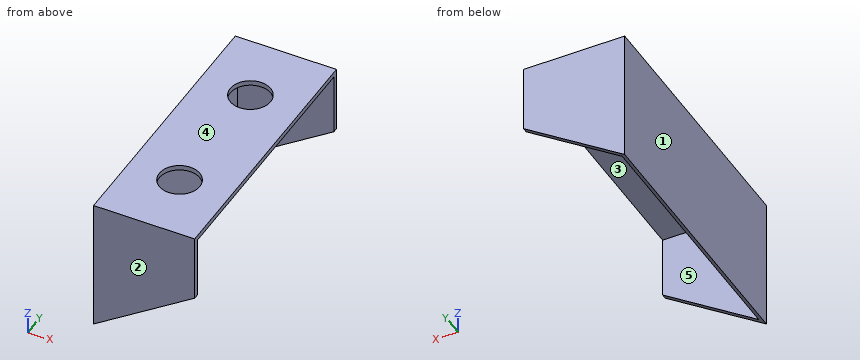
from build123d import *

# Parameters (mm, degrees)
F1_DEPTH = 50.8
F2_R     = 7.62
F3_DEPTH = 50.801
F4_T     = -1.905


with BuildPart() as f1:
    # F0 (on Front) → F1 (new body, symmetric)
    with BuildSketch(Plane.XZ):
        Polygon((0, 50.8), (0, 0), (38.1, 25.4), (38.1, 50.8), align=None)
    extrude(amount=F1_DEPTH, both=True)

    # F2 (on face) → F3 (cut, through all)
    with BuildSketch(Plane.XY.offset(50.8)):
        with Locations((19.05, 25.4)):
            Circle(F2_R)
        with Locations((19.05, -25.4)):
            Circle(F2_R)
    extrude(amount=-F3_DEPTH, mode=Mode.SUBTRACT)

    # F4
    f4_openings = [f1.faces().sort_by_distance(p)[0] for p in [
        (19.05, 0, 12.7),
        (38.1, 0, 38.1),
        (11.43, -25.4, 29.104782),
        (11.43, 25.4, 29.104782),
    ]]
    offset(amount=F4_T, openings=f4_openings)


solid = f1.part
Could you check a few things on this model? Use its own coordinates, in mm. Face numbers are marked on the shaded views. A direction names the side the tool comes from. Give positions to 0.01 mm unless a question says otherwise; leave off trailing zeros. Order: outer loops, then holes, each group sorted by start corner. A loop starts at its lowest first (then second) coordinate and runs counter-clockwise, first axis right, second up. Notation, with made-up numbers: (9.5, 21.5) - (27.5, 21.5) arc R17 ccw to (27.5, 36.5) - close; hole circle Ø3 at (45, 10.25). An arc over 180 degrees is marked (long way). One line per question, with ' | ' between items. Start each with the question number.
Item 1: For the marked faces 4 and 5, which set-ups out of +Z, -Z, +X, -X, +Y, -Y let a thin tool reach every point of the face, with its end or its side?
Item 2: Thinking about a two-plate mould opening in Y: for the marked faces 1, 2 and 3, which applies, pulls with the +Y half, pulls with the -Y half, needs draft (parallel to the pull), parting line crosses it, or undercut?
Item 3: I need wall thicknesses on probe 1 along Y at (x, z) = (19.05, 49.6); probe 2 along Y at (x, z) = (7.5, 46) (3 decimals); probe 3 along X at (y, z) = (25, 49). Which ranges of each line are inside material? Lowest first, please. Write a range as [from, to].
Item 4: I want a section at A-A on x = 19.05. Write out the boundary of the cut face in (y, z) (3 decimals), then the cut area to 3 significant figures.
Item 5: I'm going to push flat-ended pins straight in: pin 1 Ø3 at (x, z) = (34, 20) entering from +Y; pin 2 Ø2 at (y, z) = (15, 44) entering from +X (3 decimals). Where does each tip first touch, or does it pass through?
Item 6: I want a section at D-D on y = -23.5. Write out the boundary of the cut face in (x, z) (3 decimals).
Item 7: I want a section at C-C on x = 31.5. Write out the boundary of the cut face in (y, z) (3 decimals).
Item 8: I want a section at B-B on y = 25.4. Write out the boundary of the cut face in (x, z) (3 decimals).
Verdict:
1) face 4: +Z, +X, -X, +Y, -Y | face 5: -Z, +X
2) face 1: needs draft | face 2: pulls with the -Y half | face 3: undercut
3) probe 1: [-50.8, -33.02], [-17.78, 17.78], [33.02, 50.8] | probe 2: [-50.8, -48.895], [48.895, 50.8] | probe 3: [0, 11.44], [26.66, 38.1]
4) outline: (-50.8, 12.7) - (-48.895, 12.7) - (-48.895, 48.895) - (-33.02, 48.895) - (-33.02, 50.8) - (-50.8, 50.8) - close; (-17.78, 48.895) - (17.78, 48.895) - (17.78, 50.8) - (-17.78, 50.8) - close; (33.02, 48.895) - (48.895, 48.895) - (48.895, 12.7) - (50.8, 12.7) - (50.8, 50.8) - (33.02, 50.8) - close | area: 273 mm^2
5) pin 1: through | pin 2: x = 1.905
6) outline: (0, 0) - (1.905, 1.27) - (1.905, 48.895) - (11.671, 48.895) - (11.671, 50.8) - (0, 50.8) - close; (26.429, 48.895) - (38.1, 48.895) - (38.1, 50.8) - (26.429, 50.8) - close
7) outline: (-50.8, 21) - (-48.895, 21) - (-48.895, 48.895) - (48.895, 48.895) - (48.895, 21) - (50.8, 21) - (50.8, 50.8) - (-50.8, 50.8) - close
8) outline: (0, 0) - (1.905, 1.27) - (1.905, 48.895) - (11.43, 48.895) - (11.43, 50.8) - (0, 50.8) - close; (26.67, 48.895) - (38.1, 48.895) - (38.1, 50.8) - (26.67, 50.8) - close
